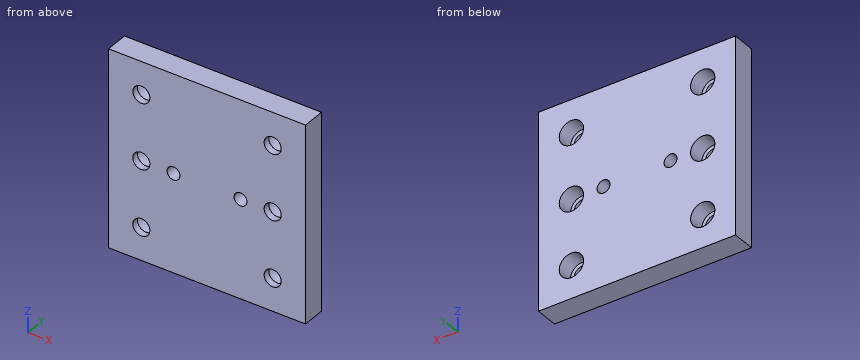
```python
from build123d import *

# Parameters (mm, degrees)
SKETCH1_W                       = 76.2
SKETCH1_H                       = 76.2
BOSS_EXTRUDE1_DEPTH             = 8.89
TAP_DRILL_FOR_M6X1_0_TAP1_D     = 5
TAP_DRILL_FOR_M6X1_0_TAP1_DEPTH = 8.89
TAP_DRILL_FOR_M6X1_0_TAP1_TIP   = 1.502151548
CBORE_FOR_M6_SHCS1_D            = 6.6
CBORE_FOR_M6_SHCS1_DEPTH        = 8.89
CBORE_FOR_M6_SHCS1_CBORE_D      = 9.4
CBORE_FOR_M6_SHCS1_CBORE_DEPTH  = 6.3
CBORE_FOR_M6_SHCS1_TIP          = 1.982840043


with BuildPart() as part:
    # Sketch1 → Boss-Extrude1 (new body)
    with BuildSketch(Plane(origin=(0, 0, 0), x_dir=(1, 0, 0), z_dir=(0, 1, 0))):
        Rectangle(SKETCH1_W, SKETCH1_H)
    extrude(amount=BOSS_EXTRUDE1_DEPTH)

    # Tap Drill for M6x1.0 Tap1
    with Locations(Plane(origin=(0, 8.89, 0), x_dir=(1, 0, 0), z_dir=(0, 1, 0))):
        with Locations((-12.954, 0), (12.954, 0)):
            Hole(TAP_DRILL_FOR_M6X1_0_TAP1_D / 2, depth=TAP_DRILL_FOR_M6X1_0_TAP1_DEPTH)
            with Locations((0, 0, -(TAP_DRILL_FOR_M6X1_0_TAP1_DEPTH + TAP_DRILL_FOR_M6X1_0_TAP1_TIP / 2))):  # 118° drill point
                Cone(0, TAP_DRILL_FOR_M6X1_0_TAP1_D / 2, TAP_DRILL_FOR_M6X1_0_TAP1_TIP, mode=Mode.SUBTRACT)

    # CBORE for M6 SHCS1
    with Locations(Plane(origin=(0, 8.89, 0), x_dir=(1, 0, 0), z_dir=(0, 1, 0))):
        with Locations((-25.4, 25.4), (25.4, 25.4), (25.4, -25.4), (-25.4, -25.4), (-25.4, 0), (25.4, 0)):
            CounterBoreHole(CBORE_FOR_M6_SHCS1_D / 2, CBORE_FOR_M6_SHCS1_CBORE_D / 2, CBORE_FOR_M6_SHCS1_CBORE_DEPTH, depth=CBORE_FOR_M6_SHCS1_DEPTH)
            with Locations((0, 0, -(CBORE_FOR_M6_SHCS1_DEPTH + CBORE_FOR_M6_SHCS1_TIP / 2))):  # 118° drill point
                Cone(0, CBORE_FOR_M6_SHCS1_D / 2, CBORE_FOR_M6_SHCS1_TIP, mode=Mode.SUBTRACT)


solid = part.part
```
CAD build for the part. Positions are in the model's coordinates, mm. Coordinates: 2 decimals unless noted, no trailing zeros. Order: outer loops, then holes, each group sorted by start corner. A loop starts at its lowest first (then second) coordinate and runs counter-clockwise, first axis right, second up.
(1) Saw through at C-C, the plane x = 25.4. Write the cut outline in (y, z).
Solution:
outline: (0, -38.1) - (8.89, -38.1) - (8.89, -30.1) - (2.59, -30.1) - (2.59, -28.7) - (0, -28.7) - close; (0, -22.1) - (2.59, -22.1) - (2.59, -20.7) - (8.89, -20.7) - (8.89, -4.7) - (2.59, -4.7) - (2.59, -3.3) - (0, -3.3) - close; (0, 3.3) - (2.59, 3.3) - (2.59, 4.7) - (8.89, 4.7) - (8.89, 20.7) - (2.59, 20.7) - (2.59, 22.1) - (0, 22.1) - close; (0, 28.7) - (2.59, 28.7) - (2.59, 30.1) - (8.89, 30.1) - (8.89, 38.1) - (0, 38.1) - close
(2) Saw through at B-B, the plane y = 1.25. Count the separate pieces of the cut face and the enclosed holes in it, and give its area (3 significant figures).
Solution:
separate pieces: 1
enclosed holes: 8
area: 5,560 mm2
(3) Pin check, flat tips, straight feed: pin 1 Ø4 at (x, z) = (25.4, 0) entering from -Y; pin 2 Ø7.5 at (x, z) = (-25.4, 25.4) entering from +Y. Stop position of each tip, or through.
Solution:
pin 1: passes through
pin 2: stops at y = 2.59
(4) Saw through at D-D, the plane z = 25.4. Write the cut outline in (x, y), and give its area (3 significant figures).
Solution:
outline: (-38.1, 0) - (-28.7, 0) - (-28.7, 2.59) - (-30.1, 2.59) - (-30.1, 8.89) - (-38.1, 8.89) - close; (-22.1, 0) - (22.1, 0) - (22.1, 2.59) - (20.7, 2.59) - (20.7, 8.89) - (-20.7, 8.89) - (-20.7, 2.59) - (-22.1, 2.59) - close; (28.7, 0) - (38.1, 0) - (38.1, 8.89) - (30.1, 8.89) - (30.1, 2.59) - (28.7, 2.59) - close
area: 525 mm2
(5) Saw through at A-A, the plane z = 0. Write the cut outline in (x, y).
Solution:
outline: (-38.1, 0) - (-28.7, 0) - (-28.7, 2.59) - (-30.1, 2.59) - (-30.1, 8.89) - (-38.1, 8.89) - close; (-22.1, 0) - (-15.45, 0) - (-15.45, 8.89) - (-20.7, 8.89) - (-20.7, 2.59) - (-22.1, 2.59) - close; (-10.45, 0) - (10.45, 0) - (10.45, 8.89) - (-10.45, 8.89) - close; (15.45, 0) - (22.1, 0) - (22.1, 2.59) - (20.7, 2.59) - (20.7, 8.89) - (15.45, 8.89) - close; (28.7, 0) - (38.1, 0) - (38.1, 8.89) - (30.1, 8.89) - (30.1, 2.59) - (28.7, 2.59) - close
(6) Drill centre lines: L1, parallel to Z at x = 25.4, y = 0.8; L2, parallel to X at y = 1, z = 25.4; L3, parallel to Z at x = -25.4, y = 6.5. Where is each one in solid material? Low to high.
Solution:
L1: z = -38.1 to -28.7, -22.1 to -3.3, 3.3 to 22.1, 28.7 to 38.1
L2: x = -38.1 to -28.7, -22.1 to 22.1, 28.7 to 38.1
L3: z = -38.1 to -30.1, -20.7 to -4.7, 4.7 to 20.7, 30.1 to 38.1
